```python
from build123d import *

# Parameters (mm, degrees)
SKETCH_1_R      = 2
EXTRUDE_1_DEPTH = 5
FILLET_1_R      = 1


with BuildPart() as part:
    # 草图1 → 凸台-拉伸1 (new body)
    with BuildSketch(Plane(origin=(0, 0, 0), x_dir=(1, 0, 0), z_dir=(0, 1, 0))):
        Polygon((-35, 5), (35, 5), (35, -5), (35, -8), (-35, -8), (-35, -5), align=None)
        with Locations(Location((-27, 0, 0), (0, 0, 270))):
            Circle(SKETCH_1_R, mode=Mode.SUBTRACT)
        with Locations(Location((-9, 0, 0), (0, 0, 270))):
            Circle(SKETCH_1_R, mode=Mode.SUBTRACT)
        with Locations(Location((9, 0, 0), (0, 0, 90))):
            Circle(SKETCH_1_R, mode=Mode.SUBTRACT)
        with Locations(Location((27, 0, 0), (0, 0, 90))):
            Circle(SKETCH_1_R, mode=Mode.SUBTRACT)
    extrude(amount=EXTRUDE_1_DEPTH)

    # 圆角1
    fillet_1_edges = [part.edges().sort_by_distance(p)[0] for p in [
        (35, 2.5, 8),
        (-35, 2.5, 8),
        (-35, 2.5, -5),
        (35, 2.5, -5),
    ]]
    fillet(fillet_1_edges, radius=FILLET_1_R)


solid = part.part
```
The model under review builds one solid part; all positions refer to its coordinate system, in mm. Give positions to 0.01 mm unless a question says otherwise; leave off trailing zeros. Write each loop counter-clockwise with the first axis right and the second up, starting at its lowest first coordinate (ties: lowest second). Pieces come first, ordered by that corner, then holes. Notation, with made-up numbers: (14, 21) -> (55, 21) arc R19 ccw to (55, 41) -> close; hole circle Ø5 at (59.25, 57). An arc over 180 degrees is marked (long way). Answer in a Markdown table with one row per item.
1) Mouldability with a two-part tool opening along X and no side actions: class faces 1 (the cylindrical face through (29, 2, 0)), 2 (the flat face through (0, 2, 8)), 3 (the flat face through (35, 2, 2)) as +X half, -X half, draft (parallel to the pull), parting line (faces both ways), or undercut.
Worked answers:
| item | result |
|---|---|
| face 1 | undercut |
| face 2 | draft |
| face 3 | +X half |
2) Clearance check with flat-ended pins moving along their axes: P1, Ø2, axis at x = 8, z = 4, coming from the -Y side; P2, Ø3.5, axis at x = -27, z = 0, coming from the -Y side. State where each tip first meets the part, or that it passes through.
Worked answers:
| item | result |
|---|---|
| P1 | y = 0 |
| P2 | through |
3) For L1, parallel to Z at x = 27, y = 3.6; L2, parallel to X at y = 1.1, z = 0; L3, parallel to X at y = 3.35, z = -1, list the stretches that pass through material, from the lowest coordinate up. Write a range as [from, to].
Worked answers:
| item | result |
|---|---|
| L1 | [-5, -2], [2, 8] |
| L2 | [-35, -29], [-25, -11], [-7, 7], [11, 25], [29, 35] |
| L3 | [-35, -28.73], [-25.27, -10.73], [-7.27, 7.27], [10.73, 25.27], [28.73, 35] |
4) Add section C-C on x = 9. State the section outline as (y, z) points.
Worked answers:
| item | result |
|---|---|
| outline | (0, -5) -> (5, -5) -> (5, -2) -> (0, -2) -> close; (0, 2) -> (5, 2) -> (5, 8) -> (0, 8) -> close |
5) Add section B-B on y = 0.9. State the section outline as (x, z) points, plus the area to 3 significant figures.
Worked answers:
| item | result |
|---|---|
| outline | (-35, -4) arc R1 ccw to (-34, -5) -> (34, -5) arc R1 ccw to (35, -4) -> (35, 7) arc R1 ccw to (34, 8) -> (-34, 8) arc R1 ccw to (-35, 7) -> close; hole circle Ø4 at (-27, 0); hole circle Ø4 at (-9, 0); hole circle Ø4 at (9, 0); hole circle Ø4 at (27, 0) |
| area | 859 mm² |
6) Add section A-A on z = 0. State the section outline as (x, y) points, plus the area to 3 significant figures.
Worked answers:
| item | result |
|---|---|
| outline | (-35, 0) -> (-29, 0) -> (-29, 5) -> (-35, 5) -> close; (-25, 0) -> (-11, 0) -> (-11, 5) -> (-25, 5) -> close; (-7, 0) -> (7, 0) -> (7, 5) -> (-7, 5) -> close; (11, 0) -> (25, 0) -> (25, 5) -> (11, 5) -> close; (29, 0) -> (35, 0) -> (35, 5) -> (29, 5) -> close |
| area | 270 mm² |
